Autodesk Inventor part; units mm, degrees
ref_plane "YZ Plane" through (0, 0, 0) normal (1, 0, 0) x (0, 1, 0)
ref_plane "XZ Plane" through (0, 0, 0) normal (0, 1, 0) x (-1, 0, 0)
ref_plane "XY Plane" through (0, 0, 0) normal (0, 0, 1) x (1, 0, 0)
sketch "Sketch1" plane through (0, 0, 0) normal (0, 0, 1) x (1, 0, 0)
  circle A0 centre (0, 0) radius 3.85
  circle A1 centre (0, 0) radius 3.125
  dimension "d0" = 7.7
  dimension "d2" = 6.25
extrude "Extrusion1" add sketch "Sketch1" along normal blind 14.45
sketch "Sketch2" plane through (0, 0, 14.45) normal (0, 0, 1) x (1, 0, 0)
  circle A0 centre (0, 0) radius 3.85
  line L0 (-2.8579, 4.95) -> (2.8579, 4.95)
  line L1 (2.8579, 4.95) -> (5.7158, 0)
  line L2 (5.7158, 0) -> (2.8579, -4.95)
  line L3 (2.8579, -4.95) -> (-2.8579, -4.95)
  line L4 (-2.8579, -4.95) -> (-5.7158, 0)
  line L5 (-5.7158, 0) -> (-2.8579, 4.95)
  dimension "d5" = 9.9
extrude "Extrusion2" add sketch "Sketch2" against normal blind 2.3
sketch "Sketch3" plane through (0, 0, 12.15) normal (0, 0, -1) x (-1, 0, 0)
  circle A0 centre (0, 0) radius 3.85
  circle A1 centre (0, 0) radius 7.4
  dimension "d8" = 14.8
extrude "Extrusion3" add sketch "Sketch3" along normal blind 1
thread "Thread1"
properties part number "TUNING PEG RETAINER"
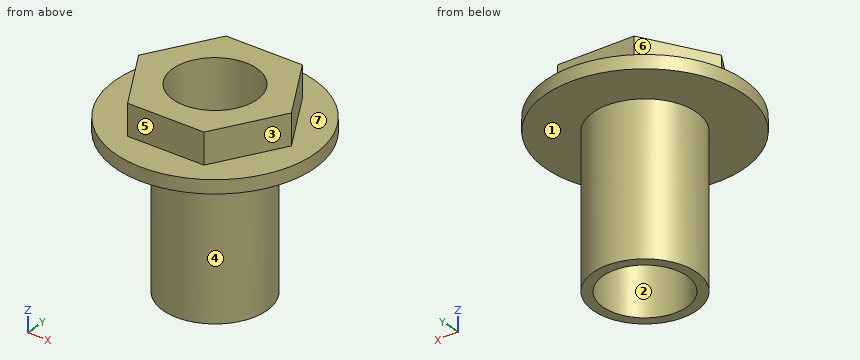
Read the model definition and answer for the solid it produces. Units are mm, in the model's axes. Face numbers are marked on the shaded views. A direction names the side the tool comes from. Give positions to 0.01 mm unless a question says otherwise; leave off trailing zeros. Order: outer loops, then holes, each group sorted by start corner. A loop starts at its lowest first (then second) coordinate and runs counter-clockwise, first axis right, second up. Notation, with made-up numbers: (-4.75, 70.25) -> (21.25, 70.25) arc R11 cw to (21.25, 76.25) -> close; hole circle Ø2 at (81, -4.75). An arc over 180 degrees is marked (long way). Write item = value, one per line.
1. A cutting plane is placed at B-B, the plane y = -1. Write down the section's boundary in (x, z), and give its area (3 significant figures).
Numbers:
outline = (-7.33, 11.15) -> (-3.72, 11.15) -> (-3.72, 0) -> (-2.96, 0) -> (-2.96, 14.45) -> (-5.14, 14.45) -> (-5.14, 12.15) -> (-7.33, 12.15) -> close; (2.96, 0) -> (3.72, 0) -> (3.72, 11.15) -> (7.33, 11.15) -> (7.33, 12.15) -> (5.14, 12.15) -> (5.14, 14.45) -> (2.96, 14.45) -> close
area = 35.6 mm²
2. A cutting plane is placed at A-A, the plane x = 0. Write down the section's boundary in (y, z) (3 decimals).
Numbers:
outline = (-7.4, 11.15) -> (-3.85, 11.15) -> (-3.85, 0) -> (-3.125, 0) -> (-3.125, 14.45) -> (-4.95, 14.45) -> (-4.95, 12.15) -> (-7.4, 12.15) -> close; (3.125, 0) -> (3.85, 0) -> (3.85, 11.15) -> (7.4, 11.15) -> (7.4, 12.15) -> (4.95, 12.15) -> (4.95, 14.45) -> (3.125, 14.45) -> close
3. Given pin 1 (1 mm diameter, centred on x = 0.5, y = 2.5, fed in from +Z); pin 2 (1.5 mm diameter, centred on x = 3, z = 13, fed in from -Y); pin 3 (3 mm diameter, centred on x = -1, z = 9, fed in from -Y); pin 4 (1.1 mm diameter, centred on x = -1, z = 13, fed in from +Y), each flat-ended and moving along its own axis, determine where each tip first touches the part or whether it passes through.
Numbers:
pin_1 = through
pin_2 = -4.95
pin_3 = -3.85
pin_4 = 4.95
4. A cutting plane is placed at D-D, the plane x = 5.25. Write down the section's boundary in (y, z), and give its area (3 significant figures).
Numbers:
outline = (-5.22, 11.15) -> (5.22, 11.15) -> (5.22, 12.15) -> (0.81, 12.15) -> (0.81, 14.45) -> (-0.81, 14.45) -> (-0.81, 12.15) -> (-5.22, 12.15) -> close
area = 14.1 mm²
5. Straight lines are drawn through the part: line 1 along Y through (x, z) = (0, 5.75) (3 decimals); line 2 along Z through (x, y) = (-5, -1); line 3 along Y through (x, z) = (-2.75, 4.5). For each, find the intervals that lie inside material, in ascending order.
Numbers:
line_1 = -3.85 to -3.125, 3.125 to 3.85
line_2 = 11.15 to 14.45
line_3 = -2.69 to -1.48, 1.48 to 2.69
6. For the marked faces 4, 5, 6 and 7, determine the directions among +Z, -Z, +X, -X, +Y, -Y from which every point of the face is accessible in a straight line to the end or side of a thin tool.
Numbers:
face_4 = -Z
face_5 = +Z, +X, -X, -Y
face_6 = +Z, -X, +Y
face_7 = +Z
7. The mould has two halves that part along X. Classify the marked faces 1, 2 and 3: +X half, -X half, draft (parallel to the pull), parting line (faces both ways), or undercut.
Numbers:
face_1 = draft
face_2 = undercut
face_3 = +X half
8. A cutting plane is placed at C-C, the plane z = 10.25. Write down the section's boundary in (x, y) (3 decimals), and give its area (3 significant figures).
Numbers:
outline = circle Ø7.7 at (0, 0); hole circle Ø6.25 at (0, 0)
area = 15.9 mm²
